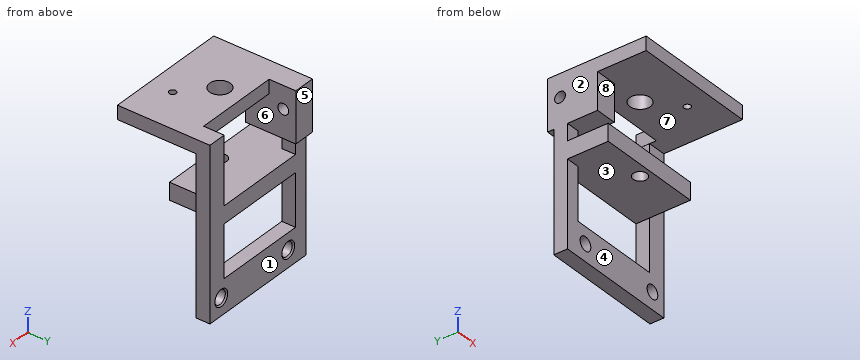
```python
from build123d import *

# Parameters (mm, degrees)
SKETCH1_R                             = 1.561475409
SKETCH1_R_2                           = 4.762499999
BOSS_EXTRUDE1_DEPTH                   = 6.35
BOSS_EXTRUDE2_DEPTH                   = 23.368
SKETCH3_W                             = 6.35
SKETCH3_H                             = 76.2
SKETCH3_W_2                           = 8.382
BOSS_EXTRUDE3_DEPTH                   = 6.35
CUT_EXTRUDE1_REACH                    = 102.468
SKETCH4_R                             = 2.5
SKETCH5_W                             = 57.15
SKETCH5_H                             = 15.458350333
BOSS_EXTRUDE4_DEPTH                   = 6.35
F_1_4_0_25_DIAMETER_HOLE1_D           = 6.35
F_1_4_0_25_DIAMETER_HOLE1_CSINK_D     = 7.62
F_1_4_0_25_DIAMETER_HOLE1_CSINK_ANGLE = 90
SKETCH8_W                             = 48.768
SKETCH8_H                             = 7.9375
BOSS_EXTRUDE5_DEPTH                   = 25.146
CUT_EXTRUDE2_REACH                    = 62.02
SKETCH10_R                            = 3.175


with BuildPart() as part:
    # Sketch1 → Boss-Extrude1 (new body)
    with BuildSketch(Plane.XY):
        Polygon((23.52260518, 29.069744957), (31.942128684, 29.069744957), (31.942128684, -13.602255043), (-25.207871316, -13.602255043), (-25.207871316, 8.844196721), (-25.207871316, 31.958196721), (-18.857871316, 31.958196721), (-15.310946905, 31.958196721), (-15.310946905, 22.656471706), (-15.310946905, 19.620299994), (23.52260518, 19.620299994), (23.52260518, 22.656471706), align=None)
        with Locations((12.892128684, -2.934255043)):
            Circle(SKETCH1_R, mode=Mode.SUBTRACT)
        with Locations((6.7e-08, 8.844196721)):
            Circle(SKETCH1_R_2, mode=Mode.SUBTRACT)
    extrude(amount=-BOSS_EXTRUDE1_DEPTH)

    # Sketch2 → Boss-Extrude2 (add)
    with BuildSketch(Plane.XY):
        Polygon((-15.310946905, 31.958196721), (-18.857871316, 31.958196721), (-25.207871316, 31.958196721), (-25.207871316, 8.844196721), (-18.857871316, 8.844196721), (-15.310946905, 8.844196721), (-15.310946905, 19.620299994), align=None)
    extrude(amount=-BOSS_EXTRUDE2_DEPTH)

    # Sketch3 → Boss-Extrude3 (add)
    with BuildSketch(Plane(origin=(0, 29.069744957, 0), x_dir=(1, 0, 0), z_dir=(0, 1, 0))):
        with Locations((-22.032871316, 38.1)):
            Rectangle(SKETCH3_W, SKETCH3_H)
        with Locations((27.751128684, 38.1)):
            Rectangle(SKETCH3_W_2, SKETCH3_H)
    extrude(amount=-BOSS_EXTRUDE3_DEPTH)

    # Sketch4 → Cut-Extrude1 (cut, up to next)
    with BuildSketch(Plane.ZY.offset(25.207871316), mode=Mode.PRIVATE) as cut_extrude1_sk1:
        with Locations(Location((-10.437499124, 26.162307082, 0), (0, 0, 270))):
            Circle(SKETCH4_R)
    cut_extrude1_tool1 = extrude(cut_extrude1_sk1.sketch, amount=-CUT_EXTRUDE1_REACH, mode=Mode.PRIVATE) & part.part
    add(cut_extrude1_tool1.solids().sort_by_distance((-25.207871, 26.162307, -10.437499))[0], mode=Mode.SUBTRACT)

    # Sketch5 → Boss-Extrude4 (add)
    with BuildSketch(Plane(origin=(0, 29.069744957, 0), x_dir=(1, 0, 0), z_dir=(0, 1, 0))):
        with Locations((3.367128684, 70.765431119)):
            Rectangle(SKETCH5_W, SKETCH5_H)
    extrude(amount=-BOSS_EXTRUDE4_DEPTH)

    # 1/4 (0.25) Diameter Hole1 (through all)
    with Locations(Plane(origin=(0, 29.069744957, 0), x_dir=(1, 0, 0), z_dir=(0, 1, 0))):
        with Locations((-14.553595262, 70.62526945), (25.19519669, 70.62526945)):
            CounterSinkHole(F_1_4_0_25_DIAMETER_HOLE1_D / 2, F_1_4_0_25_DIAMETER_HOLE1_CSINK_D / 2, counter_sink_angle=F_1_4_0_25_DIAMETER_HOLE1_CSINK_ANGLE)

    # Sketch8 → Boss-Extrude5 (add)
    with BuildSketch(Plane(origin=(0, 29.069744957, 0), x_dir=(1, 0, 0), z_dir=(0, 1, 0))):
        with Locations((-0.823871316, 35.01875)):
            Rectangle(SKETCH8_W, SKETCH8_H)
    extrude(amount=-BOSS_EXTRUDE5_DEPTH)

    # Sketch10 → Cut-Extrude2 (cut, up to next)
    with BuildSketch(Plane(origin=(0, 0, -38.9875), x_dir=(-1, 0, 0), z_dir=(0, 0, -1)), mode=Mode.PRIVATE) as cut_extrude2_sk1:
        with Locations((-6.7e-08, 8.844196721)):
            Circle(SKETCH10_R)
    cut_extrude2_tool1 = extrude(cut_extrude2_sk1.sketch, amount=-CUT_EXTRUDE2_REACH, mode=Mode.PRIVATE) & part.part
    add(cut_extrude2_tool1.solids().sort_by_distance((0, 8.844197, -38.9875))[0], mode=Mode.SUBTRACT)


solid = part.part
```
Verification items for the finished model (mm, model axes). Face numbers are marked on the shaded views. A direction names the side the tool comes from. Give positions to 0.01 mm unless a question says otherwise; leave off trailing zeros. Loops run counter-clockwise (first coordinate to the right, second up) from the corner with the lowest first, then second, coordinate; pieces in that order, holes last. Notation, with made-up numbers: M 0.25,-5.75 L 47.25,-5.75 A15 cw 47.25,2.25 Z; hole C 21.25,-10.75 d11. An arc over 180 degrees is marked long. One line per question, with ' | ' between items.
Item 1: Section check B-B, the plane z = -61.5. Record the cut outline in (x, y).
Completed:
outline: M -25.21,22.72 L -18.86,22.72 L -18.86,29.07 L -25.21,29.07 Z; M 23.56,22.72 L 31.94,22.72 L 31.94,29.07 L 23.56,29.07 Z
Item 2: Section check C-C, the plane x = 19. Record the cut outline in (y, z).
Completed:
outline: M -13.6,-6.35 L 19.62,-6.35 L 19.62,0 L -13.6,0 Z; M 3.92,-38.99 L 29.07,-38.99 L 29.07,-31.05 L 3.92,-31.05 Z; M 22.72,-78.49 L 29.07,-78.49 L 29.07,-63.04 L 22.72,-63.04 Z
Item 3: Section check D-D, the plane y = 2.5. Record the cut outline in (x, z).
Completed:
outline: M -25.21,-6.35 L 31.94,-6.35 L 31.94,0 L -25.21,0 Z
Item 4: Thickness scan on line 1 (Z direction, x = -10, y = 17); line 2 (Z direction, x = -18, y = 19); line 3 (X direction, y = 24, z = -42). Record the ranges inside material, lowest first. Write a range as [from, to].
Completed:
line 1: z = [-38.99, -31.05], [-6.35, 0] | line 2: z = [-38.99, -31.05], [-23.37, 0] | line 3: x = [-25.21, -18.86], [23.56, 31.94]
Item 5: Tool access check on the marked faces 4, 5, 6, 7 and 8. Record the directions out of +Z, -Z, +X, -X, +Y, -Y that give a thin tool (end or side, any length) a straight path to the whole face; none if there is none.
Completed:
face 4: -Z, +X, -Y | face 5: +Z, -Z, +X, -X, +Y | face 6: +Y | face 7: +X, -Y | face 8: +X, -X, -Y
Item 6: Depth check by flat-ended pin: P1, Ø6.5, axis at y = 14, z = -33.5, coming from the +X side; P2, Ø11, axis at x = -20.5, z = -19, coming from the -Y side; P3, Ø8.5, axis at x = -14.55, z = -70.63, coming from the -Y side. Enter the tip coordinate at first touch or a pass-through.
Completed:
P1: stops at x = 23.56 | P2: stops at y = 8.84 | P3: stops at y = 22.72
Item 7: Draft check along X on the marked faces 1, 2 and 3. Enter one of: +X half, -X half, draft (parallel to the pull), parting line (faces both ways), or undercut.
Completed:
face 1: draft | face 2: -X half | face 3: undercut
Item 8: Section check A-A, the plane x = 0. Record the cut outline in (y, z).
Completed:
outline: M -13.6,-6.35 L 4.08,-6.35 L 4.08,0 L -13.6,0 Z; M 3.92,-38.99 L 5.67,-38.99 L 5.67,-31.05 L 3.92,-31.05 Z; M 12.02,-38.99 L 29.07,-38.99 L 29.07,-31.05 L 12.02,-31.05 Z; M 13.61,-6.35 L 19.62,-6.35 L 19.62,0 L 13.61,0 Z; M 22.72,-78.49 L 29.07,-78.49 L 29.07,-63.04 L 22.72,-63.04 Z
